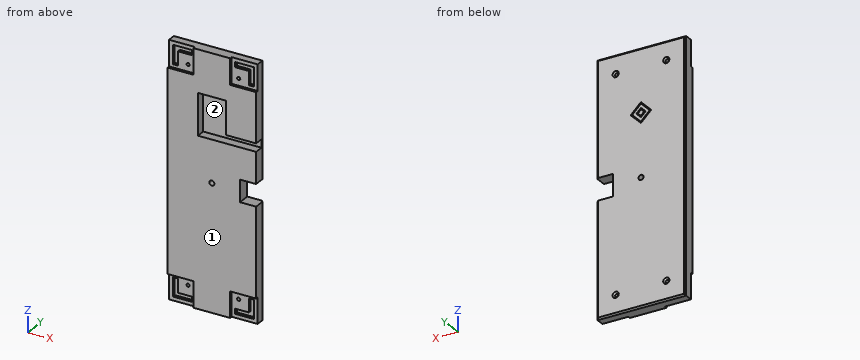
from build123d import *

# Parameters (mm, degrees)
BOSS_EXTRUDE1_DEPTH = 4
SKETCH2_W           = 140
SKETCH2_H           = 400
BOSS_EXTRUDE2_DEPTH = 15.05
SKETCH3_W           = 8
SKETCH3_H           = 22
SKETCH3_H_2         = 8
SKETCH3_W_2         = 22
SKETCH3_R           = 2.5
CUT_EXTRUDE1_DEPTH  = 5
CUT_EXTRUDE2_REACH  = 255.21
SKETCH4_R           = 2.5
CHAMFER1_SIZE       = 2.38
CUT_EXTRUDE3_REACH  = 255.48
SKETCH5_R           = 4
CUT_EXTRUDE4_DEPTH  = 1.75
SKETCH7_W           = 50
SKETCH7_H           = 13
CUT_EXTRUDE5_DEPTH  = 14.05
CUT_EXTRUDE6_REACH  = 255.48
SKETCH8_W           = 25.391909776
SKETCH8_H           = 34.82217309


with BuildPart() as part:
    # Sketch1 → Boss-Extrude1 (new body)
    with BuildSketch(Plane(origin=(0, -20.720705818, 0), x_dir=(1, 0, 0), z_dir=(0, 1, 0))):
        Polygon((6.005034784, -235.03386434), (6.005034784, -194.03386434), (47.005034784, -194.03386434), (47.005034784, 123.96613566), (6.005034784, 123.96613566), (6.005034784, 164.96613566), (-51.994965216, 164.96613566), (-51.994965216, 123.96613566), (-92.994965216, 123.96613566), (-92.994965216, -194.03386434), (-51.994965216, -194.03386434), (-51.994965216, -235.03386434), align=None)
    extrude(amount=-BOSS_EXTRUDE1_DEPTH)

    # Sketch2 → Boss-Extrude2 (add)
    with BuildSketch(Plane(origin=(0, -20.720705818, 0), x_dir=(1, 0, 0), z_dir=(0, 1, 0))):
        with Locations((-22.994965216, -35.03386434)):
            Rectangle(SKETCH2_W, SKETCH2_H)
    extrude(amount=BOSS_EXTRUDE2_DEPTH)

    # Sketch3 → Cut-Extrude1 (cut)
    # profile 1 of 14: a face of its own
    with BuildSketch(Plane.XZ.offset(20.720705818)):
        with Locations((37.005034784, 210.03386434)):
            Rectangle(SKETCH3_W, SKETCH3_H)
    # profile 2 of 14: a face of its own
    with BuildSketch(Plane.XZ.offset(20.720705818)):
        with Locations((37.005034784, 225.03386434)):
            Rectangle(SKETCH3_W, SKETCH3_H_2)
    # profile 3 of 14: a face of its own
    with BuildSketch(Plane.XZ.offset(20.720705818)):
        with Locations((22.005034784, 225.03386434)):
            Rectangle(SKETCH3_W_2, SKETCH3_H_2)
    # profile 4 of 14: a face of its own
    with BuildSketch(Plane.XZ.offset(20.720705818)):
        with Locations((-67.994965216, 225.03386434)):
            Rectangle(SKETCH3_W_2, SKETCH3_H_2)
    # profile 5 of 14: a face of its own
    with BuildSketch(Plane.XZ.offset(20.720705818)):
        with Locations((-82.994965216, 210.03386434)):
            Rectangle(SKETCH3_W, SKETCH3_H)
    # profile 6 of 14: a face of its own
    with BuildSketch(Plane.XZ.offset(20.720705818)):
        with Locations((-82.994965216, 225.03386434)):
            Rectangle(SKETCH3_W, SKETCH3_H_2)
        with Locations((-82.994965216, 225.03386434)):
            Circle(SKETCH3_R, mode=Mode.SUBTRACT)
    # profile 7 of 14: a face of its own
    with BuildSketch(Plane.XZ.offset(20.720705818)):
        with Locations((-82.994965216, 225.03386434)):
            Circle(SKETCH3_R)
    # profile 8 of 14: a face of its own
    with BuildSketch(Plane.XZ.offset(20.720705818)):
        with Locations((-67.994965216, -154.96613566)):
            Rectangle(SKETCH3_W_2, SKETCH3_H_2)
    # profile 9 of 14: a face of its own
    with BuildSketch(Plane.XZ.offset(20.720705818)):
        with Locations((-82.994965216, -139.96613566)):
            Rectangle(SKETCH3_W, SKETCH3_H)
    # profile 10 of 14: a face of its own
    with BuildSketch(Plane.XZ.offset(20.720705818)):
        with Locations((-82.994965216, -154.96613566)):
            Rectangle(SKETCH3_W, SKETCH3_H_2)
        with Locations((-82.994965216, -154.96613566)):
            Circle(SKETCH3_R, mode=Mode.SUBTRACT)
    # profile 11 of 14: a face of its own
    with BuildSketch(Plane.XZ.offset(20.720705818)):
        with Locations((-82.994965216, -154.96613566)):
            Circle(SKETCH3_R)
    # profile 12 of 14: a face of its own
    with BuildSketch(Plane.XZ.offset(20.720705818)):
        with Locations((37.005034784, -154.96613566)):
            Rectangle(SKETCH3_W, SKETCH3_H_2)
    # profile 13 of 14: a face of its own
    with BuildSketch(Plane.XZ.offset(20.720705818)):
        with Locations((22.005034784, -154.96613566)):
            Rectangle(SKETCH3_W_2, SKETCH3_H_2)
    # profile 14 of 14: a face of its own
    with BuildSketch(Plane.XZ.offset(20.720705818)):
        with Locations((37.005034784, -139.96613566)):
            Rectangle(SKETCH3_W, SKETCH3_H)
    extrude(amount=-CUT_EXTRUDE1_DEPTH, mode=Mode.SUBTRACT)

    # Sketch4 → Cut-Extrude2 (cut, up to next)
    with BuildSketch(Plane.XZ.offset(20.720705818), mode=Mode.PRIVATE) as cut_extrude2_sk1:
        with Locations(Location((-62.994965216, -134.96613566, 0), (0, 0, 270))):
            Circle(SKETCH4_R)
    cut_extrude2_tool1 = extrude(cut_extrude2_sk1.sketch, amount=-CUT_EXTRUDE2_REACH, mode=Mode.PRIVATE) & part.part
    # Sketch4 → Cut-Extrude2 (cut, up to next)
    with BuildSketch(Plane.XZ.offset(20.720705818), mode=Mode.PRIVATE) as cut_extrude2_sk2:
        with Locations(Location((17.005034784, -134.96613566, 0), (0, 0, 90))):
            Circle(SKETCH4_R)
    cut_extrude2_tool2 = extrude(cut_extrude2_sk2.sketch, amount=-CUT_EXTRUDE2_REACH, mode=Mode.PRIVATE) & part.part
    # Sketch4 → Cut-Extrude2 (cut, up to next)
    with BuildSketch(Plane.XZ.offset(20.720705818), mode=Mode.PRIVATE) as cut_extrude2_sk3:
        with Locations(Location((-62.994965216, 205.03386434, 0), (0, 0, 270))):
            Circle(SKETCH4_R)
    cut_extrude2_tool3 = extrude(cut_extrude2_sk3.sketch, amount=-CUT_EXTRUDE2_REACH, mode=Mode.PRIVATE) & part.part
    # Sketch4 → Cut-Extrude2 (cut, up to next)
    with BuildSketch(Plane.XZ.offset(20.720705818), mode=Mode.PRIVATE) as cut_extrude2_sk4:
        with Locations(Location((17.005034784, 205.03386434, 0), (0, 0, 270))):
            Circle(SKETCH4_R)
    cut_extrude2_tool4 = extrude(cut_extrude2_sk4.sketch, amount=-CUT_EXTRUDE2_REACH, mode=Mode.PRIVATE) & part.part
    add(cut_extrude2_tool1.solids().sort_by_distance((-62.994965, -20.720706, -134.966136))[0], mode=Mode.SUBTRACT)
    add(cut_extrude2_tool2.solids().sort_by_distance((17.005035, -20.720706, -134.966136))[0], mode=Mode.SUBTRACT)
    add(cut_extrude2_tool3.solids().sort_by_distance((-62.994965, -20.720706, 205.033864))[0], mode=Mode.SUBTRACT)
    add(cut_extrude2_tool4.solids().sort_by_distance((17.005035, -20.720706, 205.033864))[0], mode=Mode.SUBTRACT)

    # Chamfer1
    chamfer1_edges = [part.edges().sort_by_distance(p)[0] for p in [
        (17.005034784, -5.670705818, -137.46613566),
        (-62.994965216, -5.670705818, 207.53386434),
        (17.005034784, -5.670705818, 207.53386434),
        (-62.994965216, -5.670705818, -132.46613566),
        (-92.994965216, -5.670705818, 35.03386434),
        (-22.994965216, -5.670705818, 235.03386434),
        (47.005034784, -5.670705818, 35.03386434),
        (-22.994965216, -5.670705818, -164.96613566),
    ]]
    chamfer(chamfer1_edges, length=CHAMFER1_SIZE)

    # Sketch5 → Cut-Extrude3 (cut, up to next)
    with BuildSketch(Plane(origin=(0, -5.670705818, 0), x_dir=(1, 0, 0), z_dir=(0, 1, 0)), mode=Mode.PRIVATE) as cut_extrude3_sk1:
        with Locations(Location((-22.994965216, -35.03386434, 0), (0, 0, 270))):
            Circle(SKETCH5_R)
    cut_extrude3_tool1 = extrude(cut_extrude3_sk1.sketch, amount=-CUT_EXTRUDE3_REACH, mode=Mode.PRIVATE) & part.part
    add(cut_extrude3_tool1.solids().sort_by_distance((-22.994965, -5.670706, 35.033864))[0], mode=Mode.SUBTRACT)

    # Sketch6 → Cut-Extrude4 (cut)
    # profile 1 of 2: a face of its own
    with BuildSketch(Plane(origin=(0, -5.670705818, 0), x_dir=(1, 0, 0), z_dir=(0, 1, 0))):
        with BuildLine():
            Line((-38.613683649, -135.652582773), (-23.613683649, -150.652582773))
            ThreePointArc((-23.613683649, -150.652582773), (-22.994965216, -150.90886434), (-22.376246782, -150.652582773))
            Line((-22.376246782, -150.652582773), (-7.376246782, -135.652582773))
            ThreePointArc((-7.376246782, -135.652582773), (-7.119965216, -135.03386434), (-7.376246782, -134.415145906))
            Line((-7.376246782, -134.415145906), (-22.376246782, -119.415145906))
            ThreePointArc((-22.376246782, -119.415145906), (-22.994965216, -119.15886434), (-23.613683649, -119.415145906))
            Line((-23.613683649, -119.415145906), (-38.613683649, -134.415145906))
            ThreePointArc((-38.613683649, -134.415145906), (-38.869965216, -135.03386434), (-38.613683649, -135.652582773))
        make_face()
        Polygon((-9.232402083, -135.03386434), (-22.994965216, -148.796427473), (-36.757528349, -135.03386434), (-22.994965216, -121.271301207), align=None, mode=Mode.SUBTRACT)
    # profile 2 of 2: a face of its own
    with BuildSketch(Plane(origin=(0, -5.670705818, 0), x_dir=(1, 0, 0), z_dir=(0, 1, 0))):
        with BuildLine():
            Line((-22.376246782, -141.672326652), (-16.356502903, -135.652582773))
            ThreePointArc((-16.356502903, -135.652582773), (-16.100221337, -135.03386434), (-16.356502903, -134.415145906))
            Line((-16.356502903, -134.415145906), (-22.376246782, -128.395402027))
            ThreePointArc((-22.376246782, -128.395402027), (-22.994965216, -128.139120461), (-23.613683649, -128.395402027))
            Line((-23.613683649, -128.395402027), (-29.633427528, -134.415145906))
            ThreePointArc((-29.633427528, -134.415145906), (-29.889709095, -135.03386434), (-29.633427528, -135.652582773))
            Line((-29.633427528, -135.652582773), (-23.613683649, -141.672326652))
            ThreePointArc((-23.613683649, -141.672326652), (-22.994965216, -141.928608219), (-22.376246782, -141.672326652))
        make_face()
        Polygon((-22.994965216, -130.251557328), (-18.212658204, -135.03386434), (-22.994965216, -139.816171352), (-27.777272227, -135.03386434), align=None, mode=Mode.SUBTRACT)
    extrude(amount=-CUT_EXTRUDE4_DEPTH, mode=Mode.SUBTRACT)

    # Sketch7 → Cut-Extrude5 (cut)
    with BuildSketch(Plane.XZ.offset(24.720705818)):
        Polygon((-0.994965216, 115.03386434), (-0.994965216, 168.03386434), (-44.994965216, 168.03386434), (-44.994965216, 102.03386434), (-0.994965216, 102.03386434), align=None)
        with Locations((24.005034784, 108.53386434)):
            Rectangle(SKETCH7_W, SKETCH7_H)
    extrude(amount=-CUT_EXTRUDE5_DEPTH, mode=Mode.SUBTRACT)

    # Sketch8 → Cut-Extrude6 (cut, up to next)
    with BuildSketch(Plane(origin=(0, -5.670705818, 0), x_dir=(1, 0, 0), z_dir=(0, 1, 0)), mode=Mode.PRIVATE) as cut_extrude6_sk1:
        with Locations((34.309079896, -35.03386434)):
            Rectangle(SKETCH8_W, SKETCH8_H)
    cut_extrude6_tool1 = extrude(cut_extrude6_sk1.sketch, amount=-CUT_EXTRUDE6_REACH, mode=Mode.PRIVATE) & part.part
    add(cut_extrude6_tool1.solids().sort_by_distance((34.30908, -5.670706, 35.033864))[0], mode=Mode.SUBTRACT)


solid = part.part
Work out the finished part from the listing and answer in its coordinate system (mm). Face numbers are marked on the shaded views. Give positions to 0.01 mm unless a question says otherwise; leave off trailing zeros. Order: outer loops, then holes, each group sorted by start corner. A loop starts at its lowest first (then second) coordinate and runs counter-clockwise, first axis right, second up. Notation, with made-up numbers: (-30.75, 39.5) -> (-8.75, 39.5) arc R27 ccw to (-8.75, 63.5) -> close; hole circle Ø10 at (-21.5, -32). An arc over 180 degrees is marked (long way). One line per item, written item: value.
Item 1: Determine the mould class of the marked faces 1 and 2 for opening direction X: released by +X, released by -X, zero draft, split by the parting line, or undercut.
Answer sheet:
face 1: zero draft
face 2: undercut
Item 2: Flat-ended cylindrical pins translate along their axes: P1, Ø15, axis at x = -70, z = 217, coming from the -Y side; P2, Ø2, axis at y = -22, z = 210, coming from the +X side; P3, Ø4.5, axis at x = 28, y = -22.5, coming from the -Z side; P4, Ø3, axis at x = -78.5, y = -22.5, coming from the +Z side. Find the tip coordinate at first contact, or state that the pin passes through.
Answer sheet:
P1: y = -20.72
P2: x = 6.01
P3: z = -164.97
P4: z = 194.03
Item 3: Find section A-A, the plane x = 26. Give the vertices of the cut face in (y, z), plus the area to 3 significant figures.
Answer sheet:
outline: (-24.72, -123.97) -> (-20.72, -123.97) -> (-20.72, -150.97) -> (-15.72, -150.97) -> (-15.72, -158.97) -> (-20.72, -158.97) -> (-20.72, -164.97) -> (-8.05, -164.97) -> (-5.67, -162.59) -> (-5.67, 17.62) -> (-24.72, 17.62) -> close; (-24.72, 52.44) -> (-5.67, 52.44) -> (-5.67, 232.65) -> (-8.05, 235.03) -> (-20.72, 235.03) -> (-20.72, 229.03) -> (-15.72, 229.03) -> (-15.72, 221.03) -> (-20.72, 221.03) -> (-20.72, 194.03) -> (-24.72, 194.03) -> (-24.72, 115.03) -> (-10.67, 115.03) -> (-10.67, 102.03) -> (-24.72, 102.03) -> close
area: 6,360 mm²
Item 4: Straight lines are drawn through the part: probe 1 along Z at (x, y) = (34.5, -11.25); probe 2 along Z at (x, y) = (20, -16.75); probe 3 along Z at (x, y) = (-69, -19.75). For each, find the intervals that lie inside material, in ascending order.
Answer sheet:
probe 1: -164.97 to 17.62, 52.44 to 102.03, 115.03 to 235.03
probe 2: -164.97 to -158.97, -150.97 to 102.03, 115.03 to 221.03, 229.03 to 235.03
probe 3: -164.97 to -158.97, -150.97 to 221.03, 229.03 to 235.03
